Geometry check sheet. Reference: the model listing, model coordinates, mm. Round coordinates to 2 decimals unless told otherwise and drop trailing zeros. Order: outer loops, then holes, each group sorted by start corner. A loop starts at its lowest first (then second) coordinate and runs counter-clockwise, first axis right, second up.
(1) Cross-section at A-A on x = 0. Enter the section's corners in (y, z).
(2) Cross-section at B-B on z = -0.1. Count the separate pieces of the cut face and the enclosed holes in it, and give its area (3 significant figures).
(3) Thickness scan on L1, parallel to Y at x = 9, z = -0.2. Record the ranges inside material, lowest first.
from build123d import *

# Parameters (mm, degrees)
SKETCH1_W           = 30
SKETCH1_H           = 3
SKETCH1_R           = 0.5
BOSS_EXTRUDE1_DEPTH = 0.5


with BuildPart() as part:
    # Sketch1 → Boss-Extrude1 (new body)
    with BuildSketch(Plane.XY):
        with Locations((13.5, 0)):
            Rectangle(SKETCH1_W, SKETCH1_H)
        Circle(SKETCH1_R, mode=Mode.SUBTRACT)
        with Locations((3, 0)):
            Circle(SKETCH1_R, mode=Mode.SUBTRACT)
        with Locations((6, 0)):
            Circle(SKETCH1_R, mode=Mode.SUBTRACT)
        with Locations((9, 0)):
            Circle(SKETCH1_R, mode=Mode.SUBTRACT)
        with Locations((12, 0)):
            Circle(SKETCH1_R, mode=Mode.SUBTRACT)
        with Locations((15, 0)):
            Circle(SKETCH1_R, mode=Mode.SUBTRACT)
        with Locations((18, 0)):
            Circle(SKETCH1_R, mode=Mode.SUBTRACT)
        with Locations((21, 0)):
            Circle(SKETCH1_R, mode=Mode.SUBTRACT)
        with Locations((24, 0)):
            Circle(SKETCH1_R, mode=Mode.SUBTRACT)
        with Locations((27, 0)):
            Circle(SKETCH1_R, mode=Mode.SUBTRACT)
    extrude(amount=-BOSS_EXTRUDE1_DEPTH)


solid = part.part
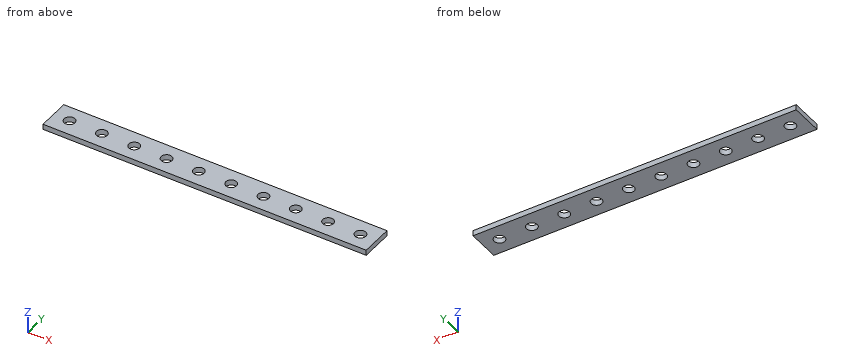
Found:
1. outline: (-1.5, -0.5) - (-0.5, -0.5) - (-0.5, 0) - (-1.5, 0) - close; (0.5, -0.5) - (1.5, -0.5) - (1.5, 0) - (0.5, 0) - close
2. separate pieces: 1
2. enclosed holes: 10
2. area: 82.1 mm2
3. L1: y = -1.5 to -0.5, 0.5 to 1.5
